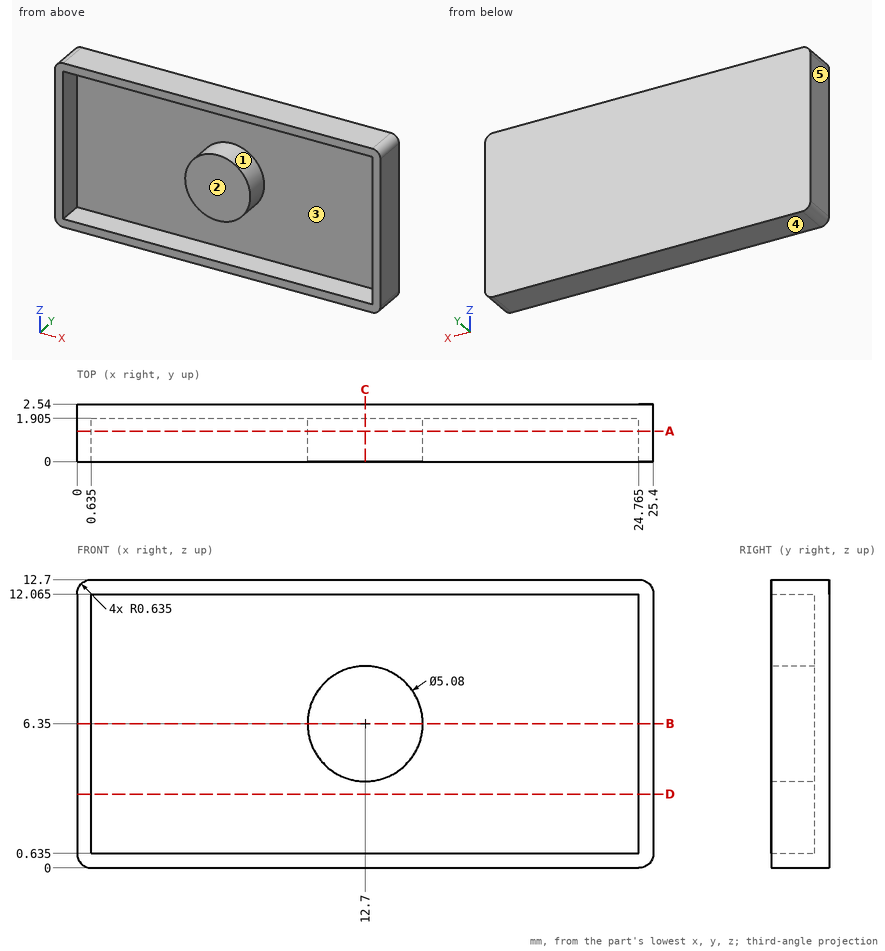
Input: dimensioned drawing with shaded views. Units: mm. Origin: part minimum x, y, z. A direction names the side the tool comes from. Give positions to 0.01 mm unless a question says otherwise; leave off trailing zeros. Write each loop counter-clockwise with the first axis right and the second up, starting at its lowest first coordinate (ties: lowest second). Pieces come first, ordered by that corner, then holes.
Q1. Section C-C, the plane x = 12.7. Output: boundary loops of the cut face in (y, z) (3 decimals).
Q2. Section A-A, the plane y = 1.35. Output: boundary loops of the cut face in (x, z) (3 decimals).
Q3. Material intervals for probe 1 along X at (y, z) = (1.7, 6.25) (3 decimals); probe 2 along X at (y, z) = (1.8, 3.25) (3 decimals); probe 3 along Z at (x, y) = (10.5, 0.15) (3 decimals), sorted ascending.
Q4. Set-up query: the marked faces 1 and 2. Return all of +Z, -Z, +X, -X, +Y, -Y with unobstructed straight access to the full face (end or side cutting, diameter ignored); none if empty.
Q5. Section B-B, the plane z = 6.35. Output: boundary loops of the cut face in (x, y) (3 decimals), plus the area to 3 significant figures.
Q6. Pull-direction query (Z, two-part tool) for the marked faces 3, 4 and 5; classes: pulls with the +Z half, pulls with the -Z half, needs draft (parallel to the pull), parting line crosses it, or undercut.
Q7. Section D-D, the plane z = 3.25. Output: boundary loops of the cut face in (x, y) (3 decimals), plus the area to 3 significant figures.
Filled in:
1. outline: (0, 0) - (2.54, 0) - (2.54, 12.7) - (0, 12.7) - (0, 12.065) - (1.905, 12.065) - (1.905, 8.89) - (0, 8.89) - (0, 3.81) - (1.905, 3.81) - (1.905, 0.635) - (0, 0.635) - close
2. outline: (0, 0.635) arc R0.635 ccw to (0.635, 0) - (24.765, 0) arc R0.635 ccw to (25.4, 0.635) - (25.4, 12.065) arc R0.635 ccw to (24.765, 12.7) - (0.635, 12.7) arc R0.635 ccw to (0, 12.065) - close; circle Ø5.08 at (12.7, 6.35); hole (0.635, 0.635) - (24.765, 0.635) - (24.765, 12.065) - (0.635, 12.065) - close
3. probe 1: x = 0 to 0.635, 10.162 to 15.238, 24.765 to 25.4
3. probe 2: x = 0 to 0.635, 24.765 to 25.4
3. probe 3: z = 0 to 0.635, 5.081 to 7.619, 12.065 to 12.7
4. face 1: -Y
4. face 2: +Z, -Z, +X, -X, -Y
5. outline: (0, 0) - (0.635, 0) - (0.635, 1.905) - (10.16, 1.905) - (10.16, 0) - (15.24, 0) - (15.24, 1.905) - (24.765, 1.905) - (24.765, 0) - (25.4, 0) - (25.4, 2.54) - (0, 2.54) - close
5. area: 28.2 mm2
6. face 3: undercut
6. face 4: pulls with the -Z half
6. face 5: needs draft
7. outline: (0, 0) - (0.635, 0) - (0.635, 1.905) - (24.765, 1.905) - (24.765, 0) - (25.4, 0) - (25.4, 2.54) - (0, 2.54) - close
7. area: 18.5 mm2
